Design review of the part shown in the three views and the two pictorial views. Dimensions are in mm from the part's minimum x, y and z. Coordinates: 2 decimals unless noted, no trailing zeros. Write each loop counter-clockwise with the first axis right and the second up, starting at its lowest first coordinate (ties: lowest second). Pieces come first, ordered by that corner, then holes. Notation, with made-up numbers: (45, 33) -> (87, 33) arc R32 cw to (87, 69) -> close; hole circle Ø6 at (-8, 43.5). An arc over 180 degrees is marked (long way). Answer in a Markdown table with one row per item. Add a question column.
Item 1: Take a section at D-D, the plane y = 46.5. Write out the cut boundary in (x, z).
Item 2: Clearance check with flat-ended pins moving along their axes: P1, Ø2.5, axis at y = 5, z = 5, coming from the +X side; P2, Ø5, axis at y = 45, z = 5, coming from the -X side. State where each tip first meets the part, or that it passes through.
Item 3: Take a section at B-B, the plane y = 5. Write out the cut boundary in (x, z), and give its area (3 significant figures).
Item 4: To check wall thickness, follow line 1 (Y direction, x = 2.75, z = 4.5); line 2 (Z direction, x = 13.5, y = 25); line 3 (Y direction, x = 18.75, z = 3.75). State the ranges of each line that lie inside material, in increasing order.
Item 5: Take a section at C-C, the plane z = 5. Write out the cut boundary in (x, y).
Item 6: Take a section at A-A, the plane x = 16.5. Write out the cut boundary in (y, z), and give its area (3 significant figures).
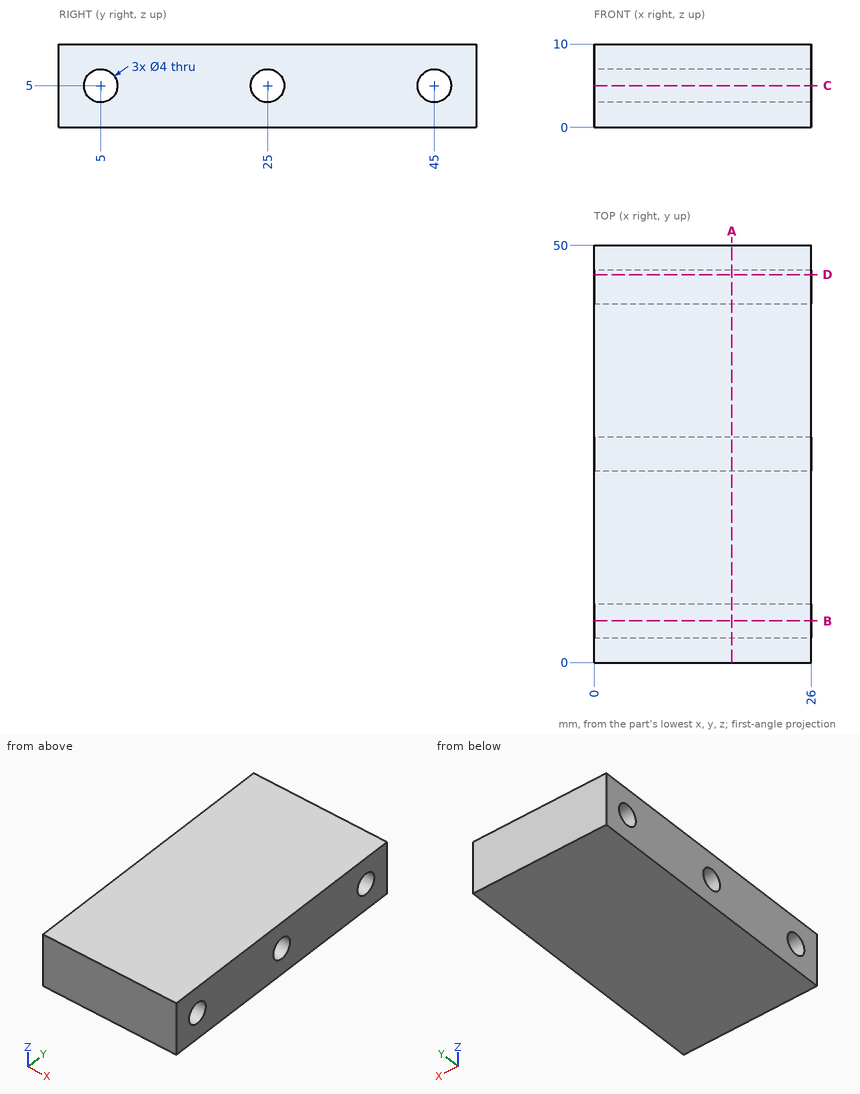
Answers:
| question | item | result |
|---|---|---|
| 1 | outline | (0, 0) -> (26, 0) -> (26, 3.68) -> (0, 3.68) -> close; (0, 6.32) -> (26, 6.32) -> (26, 10) -> (0, 10) -> close |
| 2 | P1 | passes through |
| 2 | P2 | stops at x = 0 |
| 3 | outline | (0, 0) -> (26, 0) -> (26, 3) -> (0, 3) -> close; (0, 7) -> (26, 7) -> (26, 10) -> (0, 10) -> close |
| 3 | area | 156 mm^2 |
| 4 | line 1 | y = 0 to 3.06, 6.94 to 23.06, 26.94 to 43.06, 46.94 to 50 |
| 4 | line 2 | z = 0 to 3, 7 to 10 |
| 4 | line 3 | y = 0 to 3.44, 6.56 to 23.44, 26.56 to 43.44, 46.56 to 50 |
| 5 | outline | (0, 0) -> (26, 0) -> (26, 3) -> (0, 3) -> close; (0, 7) -> (26, 7) -> (26, 23) -> (0, 23) -> close; (0, 27) -> (26, 27) -> (26, 43) -> (0, 43) -> close; (0, 47) -> (26, 47) -> (26, 50) -> (0, 50) -> close |
| 6 | outline | (0, 0) -> (50, 0) -> (50, 10) -> (0, 10) -> close; hole circle Ø4 at (5, 5); hole circle Ø4 at (25, 5); hole circle Ø4 at (45, 5) |
| 6 | area | 462 mm^2 |
